CAD build for the part. Positions are in the model's coordinates, mm. A direction names the side the tool comes from. Coordinates: 2 decimals unless noted, no trailing zeros. Write each loop counter-clockwise with the first axis right and the second up, starting at its lowest first coordinate (ties: lowest second). Pieces come first, ordered by that corner, then holes.
```python
from build123d import *

# Parameters (mm, degrees)
SKETCH_1_R               = 26
EXTRUDE_1_DEPTH          = 5
SKETCH_2_R               = 2.05
CUT_EXTRUDE_1_DEPTH      = 38.107950631
PATTERN_CIRCULAR_1_COUNT = 4
SKETCH_3_R               = 15
CUT_EXTRUDE_2_DEPTH      = 0.5
CUT_EXTRUDE_START        = -3
SKETCH_4_R               = 15
CUT_EXTRUDE_3_DEPTH      = 3
SKETCH_5_W               = 10
SKETCH_5_H               = 20
CUT_EXTRUDE_4_DEPTH      = 37.891733491
SKETCH_6_R               = 0.95
EXTRUDE_2_DEPTH          = 3


with BuildPart() as part:
    # 草图1 → 凸台-拉伸1 (new body)
    with BuildSketch(Plane.XY):
        Circle(SKETCH_1_R)
    extrude(amount=EXTRUDE_1_DEPTH)

    # 草图2 → 切除-拉伸1 (cut, through all)
    with BuildSketch(Plane(origin=(0, 0, 0), x_dir=(-1, 0, 0), z_dir=(0, 0, -1))):
        with Locations((0, 20)):
            Circle(SKETCH_2_R)
    cut_extrude_1 = extrude(amount=-CUT_EXTRUDE_1_DEPTH, mode=Mode.SUBTRACT)

    # 阵列(圆周)1: 切除-拉伸1 ×4 about axis
    pattern_circular_1_axis = Axis((0, 0, 0), (0, 0, 1))
    for i in range(1, PATTERN_CIRCULAR_1_COUNT):
        add(cut_extrude_1.rotate(pattern_circular_1_axis, i * 360 / PATTERN_CIRCULAR_1_COUNT), mode=Mode.SUBTRACT)

    # 草图3 → 切除-拉伸2 (cut)
    with BuildSketch(Plane(origin=(0, 0, 0), x_dir=(-1, 0, 0), z_dir=(0, 0, -1))):
        Circle(SKETCH_3_R)
    extrude(amount=-CUT_EXTRUDE_2_DEPTH, mode=Mode.SUBTRACT)

    # 草图4 → 切除-拉伸3 (cut)
    with BuildSketch(Plane.XY.offset(5).offset(CUT_EXTRUDE_START)):
        with Locations(Location((0, 0, 0), (0, 0, 180))):
            Circle(SKETCH_4_R)
    extrude(amount=CUT_EXTRUDE_3_DEPTH, mode=Mode.SUBTRACT)

    # 草图5 → 切除-拉伸4 (cut, through all)
    with BuildSketch(Plane.XY.offset(2)):
        Rectangle(SKETCH_5_W, SKETCH_5_H)
    extrude(amount=-CUT_EXTRUDE_4_DEPTH, mode=Mode.SUBTRACT)

    # 草图6 → 凸台-拉伸2 (add)
    with BuildSketch(Plane.XY.offset(2)):
        with Locations(Location((-6, 0, 0), (0, 0, 180))):
            Circle(SKETCH_6_R)
    extrude_2 = extrude(amount=EXTRUDE_2_DEPTH)

    # 镜向1: 凸台-拉伸2 across plane
    add(extrude_2.mirror(Plane(origin=(0, 0, 0), x_dir=(0, 0, 1), z_dir=(1, 0, 0))))


solid = part.part
```
Item 1: Saw through at D-D, the plane x = 20. Write the cut outline in (y, z).
Item 2: Two-plate mould, pull along X, no slides. Class faces 1 (the cylindrical face through (-20.633, -15.821, 2.465)), 2 (the flat face through (0, -10, 1)), 3 (the flat face through (6, 0, 5)): +X half, -X half, draft (parallel to the pull), parting line (faces both ways), or undercut.
Item 3: Saw through at A-A, the plane z = 2.85. Write the cut outline in (x, y), and give its area (3 significant figures).
Item 4: Flat gauge pins, fed straight in: pin 1 Ø0.8 at (y, z) = (2.5, 1.5) entering from -X; pin 2 Ø3 at (y, z) = (-20.5, 3.5) entering from -X; pin 3 Ø0.8 at (x, z) = (-1.5, 1.5) entering from +Y; pin 4 Ø2.5 at (x, y) = (0, -20) entering from +Z. Where does each tip first touch, or does it go through?
Item 5: Saw through at B-B, the plane x = 0. Write the cut outline in (y, z).
Item 6: Which spindle directions (+Z, -Z, +X, -X, +Y, -Y) get a long thin tool onto all of the face, cutting with end or side? Do faces 4 (the flat face through (-6, 0, 0.5)), 5 (the flat face through (-5, 0, 1)), 6 (the cylindrical face through (6.88, 0.36, 3.48)). Say none if no direction does.
Item 7: Saw through at C-C, the plane y = -7. Write the cut outline in (x, z), and give its area (3 significant figures).
Item 8: Wall check: line 1 along Y through (x, z) = (0, 4); line 2 along Y through (x, z) = (0, 1); line 3 along X through (y, z) = (5, 3.3). Give the ranges that are in metal, low to high.
Working result:
1. outline: (-16.61, 0) - (-2.05, 0) - (-2.05, 5) - (-16.61, 5) - close; (2.05, 0) - (16.61, 0) - (16.61, 5) - (2.05, 5) - close
2. face 1: parting line
2. face 2: undercut
2. face 3: draft
3. outline: circle Ø52 at (0, 0); circle Ø1.9 at (-6, 0); circle Ø1.9 at (6, 0); hole circle Ø4.1 at (-20, 0); hole circle Ø30 at (0, 0); hole circle Ø4.1 at (0, -20); hole circle Ø4.1 at (0, 20); hole circle Ø4.1 at (20, 0)
3. area: 1,370 mm2
4. pin 1: stops at x = -25.92
4. pin 2: stops at x = -17.75
4. pin 3: stops at y = 25.98
4. pin 4: passes through
5. outline: (-26, 0) - (-22.05, 0) - (-22.05, 5) - (-26, 5) - close; (-17.95, 0) - (-15, 0) - (-15, 0.5) - (-10, 0.5) - (-10, 2) - (-15, 2) - (-15, 5) - (-17.95, 5) - close; (10, 0.5) - (15, 0.5) - (15, 0) - (17.95, 0) - (17.95, 5) - (15, 5) - (15, 2) - (10, 2) - close; (22.05, 0) - (26, 0) - (26, 5) - (22.05, 5) - close
6. face 4: -Z
6. face 5: +Z, -Z
6. face 6: +Z
7. outline: (-25.04, 0) - (-13.27, 0) - (-13.27, 0.5) - (-5, 0.5) - (-5, 2) - (-13.27, 2) - (-13.27, 5) - (-25.04, 5) - close; (5, 0.5) - (13.27, 0.5) - (13.27, 0) - (25.04, 0) - (25.04, 5) - (13.27, 5) - (13.27, 2) - (5, 2) - close
7. area: 143 mm2
8. line 1: y = -26 to -22.05, -17.95 to -15, 15 to 17.95, 22.05 to 26
8. line 2: y = -26 to -22.05, -17.95 to -10, 10 to 17.95, 22.05 to 26
8. line 3: x = -25.51 to -14.14, 14.14 to 25.51
